Autodesk Inventor part; units mm, degrees
ref_plane "Work Plane2" through (10, 17.3205, 5.1062) normal (0.5, 0.866, 0) x (-0.866, 0.5, 0)
ref_plane "XZ Plane" through (0, 0, 0) normal (0, 1, 0) x (-1, 0, 0)
ref_plane "XY Plane" through (0, 0, 0) normal (0, 0, 1) x (1, 0, 0)
sketch "Sketch1" plane through (0, 0, 0) normal (1, 0, 0) x (0, 1, 0)
  line L0 (0, 0) -> (0, -33.1818)
  line L1 (4.5, 10.1062) -> (20, 10.1062)
  line L2 (20, 10.1062) -> (20, 0.1062)
  line L3 (20, 0.1062) -> (7.5, 0.1062)
  line L4 (7.5, 0.1062) -> (7.5, -29.8938)
  line L5 (7.5, -29.8938) -> (4.5, -29.8938)
  line L6 (4.5, -29.8938) -> (4.5, 10.1062)
  dimension "d0" = 9
  dimension "d1" = 15
  dimension "d2" = 30
  dimension "d3" = 10
  dimension "d4" = 40
revolve "Revolution1" add sketch "Sketch1" angle 360 about axis through (0, 0, 0) along (0, 0, -1)
sketch "Sketch2" plane through (0, 0, 10.1062) normal (0, 0, 1) x (1, 0, 0)
  point P0 (0, 0)
  point P1 (0, 16)
  dimension "d6" = 16
hole "Hole1" at (0, 16, 10.1062) direction (0, 0, -1) diameter 5 end through all
pattern_circular "Circular Pattern1" count 6 over 360 about axis through (0, 0, 5.1062) along (0, 0, -1) of "Hole1"
ref_plane "Work Plane2" through (10, 17.3205, 5.1062) normal (0.5, 0.866, 0) x (-0.866, 0.5, 0)
ref_plane "Work Plane1" through (0, 0, 0) normal (0.5, 0.866, 0) x (0, 0, 1)
sketch "Sketch3" plane through (10, 17.3205, 5.1062) normal (0.5, 0.866, 0) x (-0.866, 0.5, 0)
  line L0 (-20, 5) -> (20, 5)
  line L1 (-20, -5) -> (20, -5)
  line L2 (0, 5) -> (0, -5.1062)
  point P0 (0, -0.0531)
hole "Hole2" at (10, 17.3205, 5.0531) direction (-0.5, -0.866, 0) diameter 6.647 depth 20.2 tip angle 118
chamfer "Chamfer1" distance 0.2 angle 45 5 edges at (0, -20, 0.1062) (0, -20, 10.1062) (0, -4.5, 10.1062) (0, -4.5, -29.8938) (0, -7.5, -29.8938)
properties part number "CopperElectrode" material "Copper"
Input: part model. Units: mm. Frame: model coordinates. A direction names the side the tool comes from. Round coordinates to 2 decimals unless told otherwise and drop trailing zeros. Order: outer loops, then holes, each group sorted by start corner. A loop starts at its lowest first (then second) coordinate and runs counter-clockwise, first axis right, second up. Notation, with made-up numbers: (-22.75, -2) - (30.25, -2) arc R21 cw to (30.25, 21) - close; hole circle Ø3 at (61.25, -9.75). An arc over 180 degrees is marked (long way). One line per question, with ' | ' between items. Start each with the question number.
1) Contact query for flat-ended pins moving along their axis: P1, Ø2, axis at y = -7.5, z = -15.5, coming from the +X side; P2, Ø8, axis at x = 13.5, y = -8, coming from the -Z side; P3, Ø10, axis at y = -13, z = -18.5, coming from the +X side; P4, Ø5, axis at y = 7, z = 3.5, coming from the +X side. Output: stop coordinate, or through.
2) Cut plane C-C, the plane x = 0. Give the number of separate pieces and of enclosed holes in the cut face, then the cut area to 3 significant figures.
3) Cut plane A-A, the plane y = 0. Return the cut outline in (x, z), then the cut area to 3 significant figures.
4) Cut plane B-B, the plane z = -1.5. Return the cut outline in (x, y).
5) Pull-direction query (X, two-part tool) for faces 3 (the flat face through (0, 9, 0.106)), 4 (the cylindrical face through (-19.524, -4.336, 5.039)), 5 (the cylindrical face through (14.81, -10.31, 5.04)); classes: +X half, -X half, draft (parallel to the pull), parting line (faces both ways), or undercut.
6) Set-up query: faces 1 (the cylindrical face through (0.33, -7.493, -15.002)), 2 (the flat face through (-4, 4, 10.106)). Return all of +Z, -Z, +X, -X, +Y, -Y with unobstructed straight access to the full face (end or side cutting, diameter ignored); none if empty.
7) Ray query, probe 1 along X at (y, z) = (16, 7.5); probe 2 along X at (y, z) = (0, -7); probe 3 along X at (y, z) = (-8, 6.25). Return the intervals inside material, ascending.
Worked out:
1) P1: stops at x = 3.74 | P2: stops at z = 0.11 | P3: passes through | P4: stops at x = 19.49
2) separate pieces: 4 | enclosed holes: 0 | area: 383 mm^2
3) outline: (-20, 0.31) - (-19.8, 0.11) - (-7.5, 0.11) - (-7.5, -29.69) - (-7.3, -29.89) - (-4.7, -29.89) - (-4.5, -29.69) - (-4.5, 9.91) - (-4.7, 10.11) - (-19.8, 10.11) - (-20, 9.91) - close; (4.5, -29.69) - (4.7, -29.89) - (7.3, -29.89) - (7.5, -29.69) - (7.5, 0.11) - (19.8, 0.11) - (20, 0.31) - (20, 9.91) - (19.8, 10.11) - (4.7, 10.11) - (4.5, 9.91) - close | area: 490 mm^2
4) outline: circle Ø15 at (0, 0); hole circle Ø9 at (0, 0)
5) face 3: draft | face 4: parting line | face 5: undercut
6) face 1: -Z | face 2: +Z, +X, -X, +Y, -Y
7) probe 1: x = -12 to -2.5, 2.5 to 6.64, 11.83 to 12 | probe 2: x = -7.5 to -4.5, 4.5 to 7.5 | probe 3: x = -18.33 to -16.36, -11.36 to 11.36, 16.36 to 18.33
